Study the drawing (mm; zero at the part's minimum x, y, z) and answer. A direction names the side the tool comes from. Round coordinates to 2 decimals unless told otherwise and drop trailing zeros. Order: outer loops, then holes, each group sorted by start corner. A loop starts at its lowest first (then second) coordinate and runs counter-clockwise, first axis right, second up. Notation, with made-up numbers: (72, -24.75) - (124, -24.75) arc R38 cw to (124, 14.25) - close; hole circle Ø8 at (45, -37.5). An arc over 180 degrees is marked (long way). Put each result on its own line as item: value. Start each with the question number.
Q1. Each of these flat-tipped pins is pushed along its axis until it touches: pin 1 Ø3 at (x, y) = (54.5, 113.5) entering from +Z; pin 2 Ø16.5 at (x, y) = (42.5, 48) entering from +Z. Where does it stop, or does it pass through?
Q2. Find the intervals of material crossed by line 1 along Z through (x, y) = (49, 153.5); line 2 along X through (y, z) = (30.5, 51.5); line 3 along Z through (x, y) = (59, 96), in increasing order. Write a range as from..to.
Q3. Section A-A on x = 42.5 is taken. Give the vertices of the cut face in (y, z).
Q4. Section D-D on z = 70 is taken. Give the vertices of the cut face in (x, y), then the cut area to 3 significant figures.
Q5. Section B-B on z = 17.5 is taken. Give the vertices of the cut face in (x, y).
Q6. For a pull along Z with two mould halves and no side action, classify the marked faces 1, 2 and 3 as pulls with the +Z half, pulls with the -Z half, needs draft (parallel to the pull), parting line crosses it, or undercut.
Q7. Section C-C on y = 45 is taken. Give the vertices of the cut face in (x, z).
Q8. Which of the six approach directions +Z, -Z, +X, -X, +Y, -Y give full straight-line access (tool end or side, diameter ignored) to the marked faces 4, 5, 6, 7 and 8?
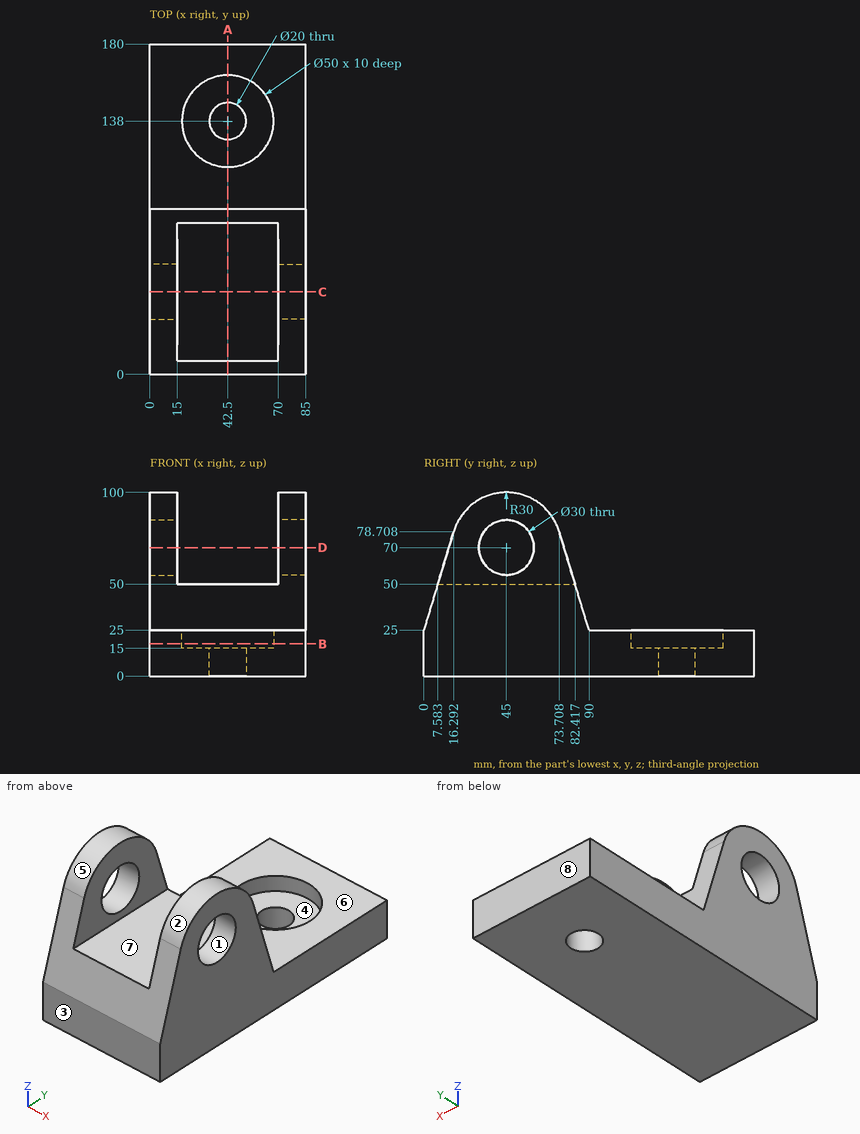
Findings:
1. pin 1: z = 25
1. pin 2: z = 50
2. line 1: 0..15
2. line 2: 0..15, 70..85
2. line 3: 0..25
3. outline: (0, 0) - (128, 0) - (128, 15) - (113, 15) - (113, 25) - (90, 25) - (82.42, 50) - (7.58, 50) - (0, 25) - close; (148, 0) - (180, 0) - (180, 25) - (163, 25) - (163, 15) - (148, 15) - close
4. outline: (0, 13.65) - (15, 13.65) - (15, 30) - (0, 30) - close; (0, 60) - (15, 60) - (15, 76.35) - (0, 76.35) - close; (70, 13.65) - (85, 13.65) - (85, 30) - (70, 30) - close; (70, 60) - (85, 60) - (85, 76.35) - (70, 76.35) - close
4. area: 981 mm2
5. outline: (0, 0) - (85, 0) - (85, 180) - (0, 180) - close; hole circle Ø50 at (42.5, 138)
6. face 1: undercut
6. face 2: pulls with the +Z half
6. face 3: needs draft
7. outline: (0, 0) - (85, 0) - (85, 55) - (70, 55) - (70, 50) - (15, 50) - (15, 55) - (0, 55) - close; (0, 85) - (15, 85) - (15, 100) - (0, 100) - close; (70, 85) - (85, 85) - (85, 100) - (70, 100) - close
8. face 4: +Z
8. face 5: +Z, +X, -X
8. face 6: +Z, +X, -X, +Y
8. face 7: +Z, +Y, -Y
8. face 8: +Z, -Z, +X, -X, +Y
